Part print with two shaded views. Sizes in mm from the minimum x, y, z corner. A direction names the side the tool comes from. Coordinates: 2 decimals unless noted, no trailing zeros. Order: outer loops, then holes, each group sorted by start corner. A loop starts at its lowest first (then second) coordinate and runs counter-clockwise, first axis right, second up.
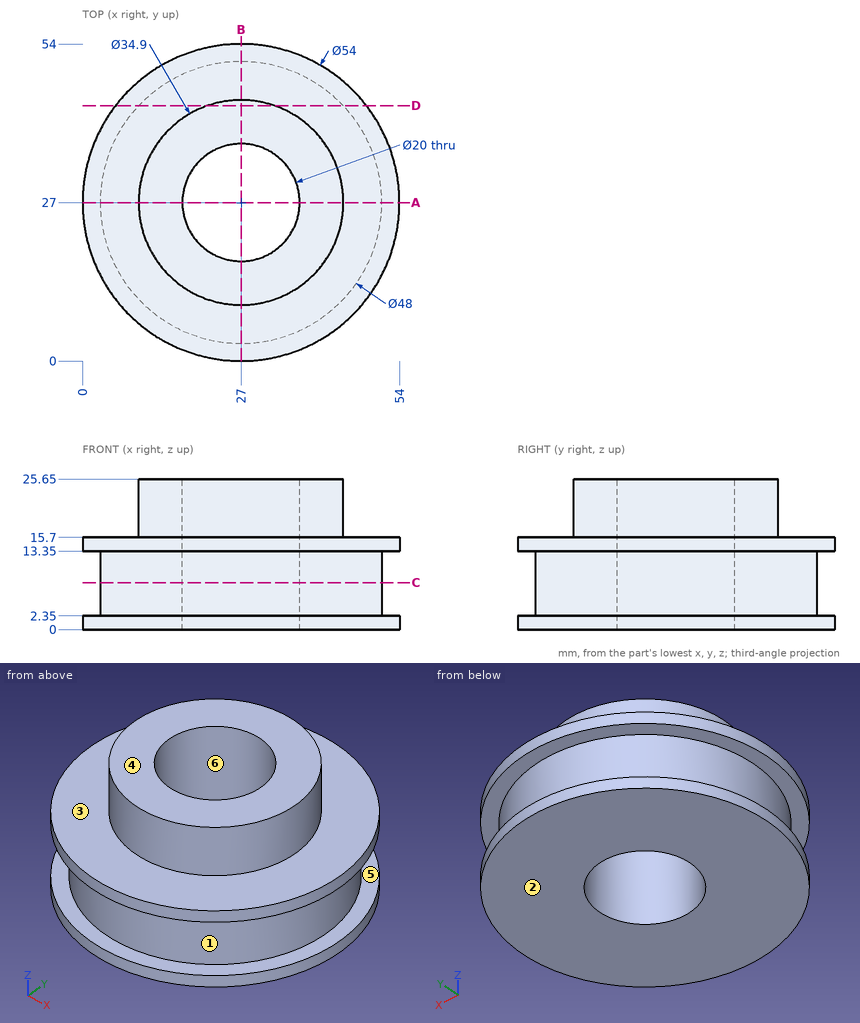
Q1. Wall check: line 1 along Y through (x, z) = (27, 16.5); line 2 along Z through (x, y) = (9, 9.5); line 3 along X through (y, z) = (27, 11.5). Give the ranges that are in metal, low to high.
Results list:
line 1: y = 9.55 to 17, 37 to 44.45
line 2: z = 0 to 2.35, 13.35 to 15.7
line 3: x = 3 to 17, 37 to 51
Q2. Cut at A-A on y = 27. Write the cut outline in (x, z), and give its area (3 significant figures).
Results list:
outline: (0, 0) - (17, 0) - (17, 25.65) - (9.55, 25.65) - (9.55, 15.7) - (0, 15.7) - (0, 13.35) - (3, 13.35) - (3, 2.35) - (0, 2.35) - close; (37, 0) - (54, 0) - (54, 2.35) - (51, 2.35) - (51, 13.35) - (54, 13.35) - (54, 15.7) - (44.45, 15.7) - (44.45, 25.65) - (37, 25.65) - close
area: 616 mm2
Q3. Pin check, flat tips, straight feed: pin 1 Ø3 at (x, y) = (10, 11.5) entering from +Z; pin 2 Ø2 at (y, z) = (45, 13.5) entering from -X; pin 3 Ø4 at (x, z) = (20.5, 19) entering from -Y; pin 4 Ø1 at (y, z) = (46.5, 16.5) entering from +X. Stop position of each tip, or through.
Results list:
pin 1: stops at z = 15.7
pin 2: stops at x = 6.02
pin 3: stops at y = 10.14
pin 4: passes through
Q4. Cut at D-D on y = 43.5. Write the cut outline in (x, z), and give its area (3 significant figures).
Results list:
outline: (5.63, 0) - (48.37, 0) - (48.37, 2.35) - (44.43, 2.35) - (44.43, 13.35) - (48.37, 13.35) - (48.37, 15.7) - (32.68, 15.7) - (32.68, 25.65) - (21.32, 25.65) - (21.32, 15.7) - (5.63, 15.7) - (5.63, 13.35) - (9.57, 13.35) - (9.57, 2.35) - (5.63, 2.35) - close
area: 697 mm2
Q5. Mould opens along Z. For the marked faces 4, 5 and 6 say: pulls with the +Z half, pulls with the -Z half, needs draft (parallel to the pull), parting line crosses it, or undercut.
Results list:
face 4: pulls with the +Z half
face 5: undercut
face 6: needs draft
Q6. Which spindle directions (+Z, -Z, +X, -X, +Y, -Y) get a long thin tool onto all of the face, cutting with end or side? Do the marked faces 1, 2 and 3. Say none if no direction does.
Results list:
face 1: none
face 2: -Z, +X, -X, +Y, -Y
face 3: +Z
Q7. Cut at C-C on z = 8. Write the cut outline in (x, y), and give its area (3 significant figures).
Results list:
outline: circle Ø48 at (27, 27); hole circle Ø20 at (27, 27)
area: 1,500 mm2
